The listing builds one solid part. Answer for the finished solid, in the listing's coordinates (mm). Face numbers are marked on the shaded views. A direction names the side the tool comes from. Round coordinates to 2 decimals unless told otherwise and drop trailing zeros. Loops run counter-clockwise (first coordinate to the right, second up) from the corner with the lowest first, then second, coordinate; pieces in that order, holes last. Notation, with made-up numbers: (23.25, 24.25) -> (34.25, 24.25) arc R10 ccw to (34.25, 40.25) -> close; hole circle Ø11 at (30, 86). An arc over 180 degrees is marked (long way). Use a Markdown table: item, result. Add a question column.
Q1. Section B-B on x = 0 is taken. Give the vertices of the cut face in (y, z), then the cut area to 3 significant figures.
Q2. Which of the six approach directions +Z, -Z, +X, -X, +Y, -Y give full straight-line access (tool end or side, diameter ignored) to the marked faces 1, 2 and 3?
Q3. For a pull along Z with two mould halves and no side action, classify the marked faces 4, 5, 6 and 7 as released by +Z, released by -Z, zero draft, split by the parting line, or undercut.
Q4. Section D-D on y = -11 is taken. Give the vertices of the cut face in (x, z), then the cut area to 3 significant figures.
Q5. Consider line 1 (Z direction, x = 0, y = -7.25); line 2 (Z direction, x = 0, y = 13.65); line 3 (X direction, y = 22, z = 28.5). Determine where each line is inside the solid, lowest interval first.
Q6. Section C-C on z = 27.5 is taken. Give the vertices of the cut face in (x, y).
Q7. Section A-A on z = 8 is taken. Give the vertices of the cut face in (x, y).
Q8. Given pin 1 Ø6 at (y, z) = (29, 10.5) entering from -X; pin 2 Ø6 at (y, z) = (-4, 30.5) entering from +X; pin 3 Ø14 at (x, y) = (32.5, 29.5) entering from -Z, each flat-ended and moving along its own axis, determine where each tip first touches the part or whether it passes through.
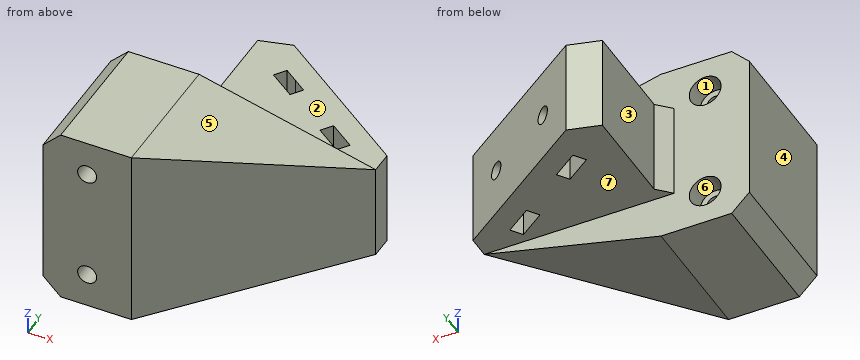
Autodesk Fusion 360 part; units mm, degrees
sketch "Sketch1" plane through (0, 0, 0) normal (0, 0, 1) x (1, 0, 0) in component "Spool Holder"
  line L0 (10, 15) -> (-10, 15)
  line L1 (-10, 15) -> (-10, -15)
  line L2 (-10, -15) -> (10, -15)
  line L3 (10, -15) -> (10, 15)
  line L4 (10, 15) -> (-10, -15) construction
  line L5 (-10, 15) -> (10, -15) construction
  line L6 (10, 15) -> (50, 15)
  line L7 (50, 15) -> (50, 20)
  line L8 (50, 20) -> (17.2339, 42.9431)
  line L9 (50, 20) -> (46.0037, 20) construction
  line L10 (50, 15) -> (10, -15)
  line L11 (17.2339, 42.9431) -> (10, 32.612)
  line L12 (17.2339, 42.9431) -> (32.2339, 42.9431) construction
  line L13 (10, 15) -> (10, 32.612)
  line L14 (10, 32.612) -> (10, 41)
  line L15 (10, 41) -> (17.2339, 42.9431)
  dimension "d1" = 30
  dimension "d2" = 20
  dimension "d3" = 40
  dimension "d4" = 5
  dimension "d5" = 145
  dimension "d6" = 40
  dimension "d7" = 125
extrude "Extrude1" add sketch "Sketch1" along normal blind 42 in component "Spool Holder"
sketch "Sketch2" plane through (0, 0, 42) normal (0, 0, 1) x (-1, 0, 0) in component "Spool Holder"
  line L0 (10, -15) -> (10, 15)
  line L1 (10, 15) -> (-10, 15)
  line L2 (-10, 15) -> (-50, -15)
  line L3 (-50, -15) -> (-50, -20)
  line L4 (-50, -20) -> (-17.2339, -42.9431)
  line L5 (-10, -41) -> (-10, -15)
  line L6 (-10, -15) -> (10, -15)
  line L7 (-10, -15) -> (-50, -15)
  line L8 (-17.2339, -42.9431) -> (-10, -41)
extrude "Extrude2" cut sketch "Sketch2" against normal blind 10 contours L3 L4 L5 L7 L8 in component "Spool Holder"
sketch "Sketch3" plane through (0, 0, 0) normal (0, 0, -1) x (1, 0, 0) in component "Spool Holder"
  line L0 (-10, 15) -> (-10, -15)
  line L1 (-10, -15) -> (10, -15)
  line L2 (10, -15) -> (10, -41)
  line L3 (17.2339, -42.9431) -> (50, -20)
  line L4 (50, -20) -> (50, -15)
  line L5 (50, -15) -> (10, 15)
  line L6 (10, 15) -> (-10, 15)
  line L7 (10, -15) -> (50, -15)
  line L8 (10, -41) -> (17.2339, -42.9431)
extrude "Extrude3" cut sketch "Sketch3" against normal blind 10 contours L2 L3 L4 L7 L8 in component "Spool Holder"
sketch "Sketch4" plane through (0, 15, 0) normal (0, 1, 0) x (-1, 0, 0) in component "Spool Holder"
  line L0 (-50, 0) -> (10, 0)
  line L1 (10, 0) -> (10, 42)
  line L2 (10, 42) -> (-50, 42)
  line L3 (-50, 42) -> (-50, 32)
  line L4 (-50, 32) -> (-10, 32)
  line L5 (-10, 32) -> (-10, 10)
  line L6 (-10, 10) -> (-50, 10)
  line L7 (-50, 10) -> (-50, 0)
  line L8 (-10, 32) -> (-10, 42)
  line L9 (-10, 10) -> (-10, 0)
  line L10 (-10, 42) -> (-50, 32)
  line L11 (-10, 0) -> (-50, 10)
  point P0 (-10, 0)
extrude "Extrude4" cut sketch "Sketch4" along normal up to surface contours L0 L7 L11 | L2 L3 L10 end surface through (50, 15, 0) normal (0.6, -0.8, 0) offset 0 in component "Spool Holder"
sketch "Sketch5" plane through (0, 0, 32) normal (0, 0, 1) x (-1, 0, 0) in component "Spool Holder"
  line L0 (-10, -15) -> (-50, -15)
  line L1 (-50, -15) -> (-50, -20)
  line L2 (-50, -20) -> (-17.2339, -42.9431)
  line L3 (-10, -41) -> (-10, -15)
  line L4 (-17.2339, -42.9431) -> (-14.366, -38.8473) construction
  line L5 (-14.366, -38.8473) -> (-54.355, -10.8467) construction
  line L6 (-14.366, -38.8473) -> (-12.5879, -36.3079) construction
  line L7 (-12.5879, -36.3079) -> (-56.8094, -5.3437) construction
  line L8 (-50, -20) -> (-45.354, -13.3649) construction
  line L9 (-50, -20) -> (-58.1, -20) construction
  line L10 (-14.366, -38.8473) -> (-22.5576, -33.1115) construction
  line L11 (-22.5576, -33.1115) -> (-20.7795, -30.5722) construction
  line L12 (-47.1321, -15.9042) -> (-38.9406, -21.64) construction
  line L13 (-38.9406, -21.64) -> (-37.1625, -19.1006) construction
  line L14 (-22.5576, -33.1115) -> (-25.4655, -31.0753)
  line L15 (-25.4655, -31.0753) -> (-23.6875, -28.536)
  line L16 (-22.5576, -33.1115) -> (-19.6496, -35.1477)
  line L17 (-19.6496, -35.1477) -> (-17.8715, -32.6084)
  line L18 (-23.6875, -28.536) -> (-17.8715, -32.6084)
  line L19 (-38.9406, -21.64) -> (-41.8486, -19.6038)
  line L20 (-41.8486, -19.6038) -> (-40.0705, -17.0644)
  line L21 (-38.9406, -21.64) -> (-36.0326, -23.6762)
  line L22 (-36.0326, -23.6762) -> (-34.2545, -21.1368)
  line L23 (-40.0705, -17.0644) -> (-34.2545, -21.1368)
  line L24 (-17.2339, -42.9431) -> (-10, -41)
  dimension "d17" = 5
  dimension "d18" = 3.1
  dimension "d19" = 125
  dimension "d20" = 8.1
  dimension "d21" = 10
  dimension "d22" = 10
  dimension "d23" = 3.55
  dimension "d24" = 3.55
  dimension "d25" = 3.55
  dimension "d26" = 3.55
extrude "Extrude5" cut sketch "Sketch5" against normal up to surface (22 mm away) contours L14 L15 L16 L17 L18 | L19 L20 L21 L22 L23 in component "Spool Holder"
sketch "Sketch6" plane through (25.8464, 36.9125, 0) normal (0.5736, 0.8192, 0) x (-0.8192, 0.5736, 0) in component "Spool Holder"
  line L0 (-29.4861, 10) -> (10.5139, 10)
  line L1 (10.5139, 32) -> (-29.4861, 32)
  line L2 (-29.4861, 32) -> (-29.4861, 10)
  line L3 (10.5139, 10) -> (10.5139, 32) construction
  line L4 (10.5139, 21) -> (-29.4861, 21) construction
  line L5 (10.5139, 21) -> (0.5139, 21) construction
  line L6 (-29.4861, 21) -> (-19.4861, 21) construction
  circle A0 centre (0.5139, 21) radius 2
  circle A1 centre (-19.4861, 21) radius 2
  line L7 (10.5139, 10) -> (10.5139, 32)
  dimension "d29" = 10
  dimension "d30" = 10
  dimension "d31" = 4
  dimension "d32" = 4
extrude "Extrude6" cut sketch "Sketch6" against normal blind 11 contours A0 | A1 in component "Spool Holder"
sketch "Sketch7" plane through (0, 15, 0) normal (0, 1, 0) x (-1, 0, 0) in component "Spool Holder"
  line L0 (-10, 42) -> (-50, 32)
  line L1 (-50, 32) -> (-10, 32)
  line L2 (-10, 32) -> (-10, 10)
  line L3 (-10, 10) -> (-50, 10)
  line L4 (-50, 10) -> (-10, 0)
  line L5 (-10, 0) -> (10, 0)
  line L6 (10, 0) -> (10, 42)
  line L7 (10, 42) -> (-10, 42)
  line L8 (-10, 42) -> (-10, 0) construction
  line L9 (-10, 42) -> (10, 42) construction
  line L10 (0, 42) -> (0, 0) construction
  line L11 (0, 42) -> (0, 34) construction
  line L12 (0, 0) -> (0, 8) construction
  circle A0 centre (0, 34) radius 3.6
  circle A1 centre (0, 8) radius 3.6
  dimension "d35" = 8
  dimension "d36" = 8
  dimension "d37" = 7.2
  dimension "d38" = 7.2
extrude "Extrude7" cut sketch "Sketch7" against normal blind 4.8 contours A0 | A1 in component "Spool Holder"
sketch "Sketch8" plane through (0, 15, 0) normal (0, 1, 0) x (-1, 0, 0) in component "Spool Holder"
  circle A0 centre (0, 8) radius 3.6
  circle A1 centre (0, 34) radius 3.6
  line L0 (-10, 42) -> (-50, 32)
  line L1 (-50, 32) -> (-10, 32)
  line L2 (-10, 32) -> (-10, 10)
  line L3 (-10, 10) -> (-50, 10)
  line L4 (-50, 10) -> (-10, 0)
  line L5 (-10, 0) -> (10, 0)
  line L6 (10, 0) -> (10, 42)
  line L7 (10, 42) -> (-10, 42)
  circle A2 centre (0, 8) radius 2.15
  circle A3 centre (0, 34) radius 2.15
  dimension "d41" = 4.3
  dimension "d42" = 4.3
extrude "Extrude8" cut sketch "Sketch8" against normal up to surface (30 mm away) contours A2 | A3 in component "Spool Holder"
chamfer "Chamfer1" distance 4 angle 45 2 edges at (-10, 0, 0) (-10, 0, 42) in component "Spool Holder"
chamfer "Chamfer2" distance 3 angle 45 1 edges at (10, 15, 21) in component "Spool Holder"
component "Spool Holder" placed x (1, 0, 0) y (0, 1, 0) z (0, 0, 1) at (0, 0, 0)
equation "d23 = ( 7.1 / 2 ) * 1 mm"
equation "d24 = ( 7.1 / 2 ) * 1 mm"
equation "d25 = ( 7.1 / 2 ) * 1 mm"
equation "d26 = ( 7.1 / 2 ) * 1 mm"
Checked values:
| question | item | result |
|---|---|---|
| 1 | outline | (-15, 0) -> (15, 0) -> (15, 4.4) -> (10.2, 4.4) -> (10.2, 5.85) -> (-15, 5.85) -> close; (-15, 10.15) -> (10.2, 10.15) -> (10.2, 11.6) -> (15, 11.6) -> (15, 30.4) -> (10.2, 30.4) -> (10.2, 31.85) -> (-15, 31.85) -> close; (-15, 36.15) -> (10.2, 36.15) -> (10.2, 37.6) -> (15, 37.6) -> (15, 42) -> (-15, 42) -> close |
| 1 | area | 974 mm2 |
| 2 | face 1 | +Y |
| 2 | face 2 | +Z, +X, -X, +Y |
| 2 | face 3 | +Z, -Z, -X, +Y |
| 3 | face 4 | zero draft |
| 3 | face 5 | released by +Z |
| 3 | face 6 | undercut |
| 3 | face 7 | released by -Z |
| 4 | outline | (-10, 4) -> (-6, 0) -> (10, 0) -> (15.33, 1.33) -> (15.33, 40.67) -> (10, 42) -> (-6, 42) -> (-10, 38) -> close; hole circle Ø4.3 at (0, 8); hole circle Ø4.3 at (0, 34) |
| 4 | area | 1,010 mm2 |
| 5 | line 1 | z = 0 to 5.85, 10.15 to 31.85, 36.15 to 42 |
| 5 | line 2 | z = 0 to 4.4, 11.6 to 30.4, 37.6 to 42 |
| 5 | line 3 | x = 10 to 34.86, 38.43 to 47.14 |
| 6 | outline | (-10, -15) -> (10, -15) -> (50, 15) -> (50, 20) -> (17.23, 42.94) -> (10, 41) -> (10, 18) -> (7, 15) -> (-10, 15) -> close; hole (17.87, 32.61) -> (23.69, 28.54) -> (25.47, 31.08) -> (22.56, 33.11) -> (19.65, 35.15) -> close; hole (34.25, 21.14) -> (40.07, 17.06) -> (41.85, 19.6) -> (36.03, 23.68) -> close |
| 7 | outline | (-10, -15) -> (-2.15, -15) -> (-2.15, 10.2) -> (-3.6, 10.2) -> (-3.6, 15) -> (-10, 15) -> close; (2.15, -15) -> (10, -15) -> (42, 9) -> (42, 15) -> (3.6, 15) -> (3.6, 10.2) -> (2.15, 10.2) -> close |
| 8 | pin 1 | stops at x = 10 |
| 8 | pin 2 | stops at x = 28.67 |
| 8 | pin 3 | stops at z = 10 |
